The listing builds one solid part. Answer for the finished solid, in the listing's coordinates (mm). A direction names the side the tool comes from. Coordinates: 2 decimals unless noted, no trailing zeros. Order: outer loops, then holes, each group sorted by start corner. A loop starts at its lowest first (then second) coordinate and runs counter-clockwise, first axis right, second up. Notation, with made-up numbers: (-2, 83) -> (41, 83) arc R8 cw to (41, 87) -> close; hole circle Ø4 at (13, -2). An arc over 180 degrees is marked (long way). Write each question's results on one line, items separated by ' | '. Start each with the question number.
(1) A tool of negligible diameter and unlimited length cuts with its end or side. For faces 1 (the face through (-2, -112, 2)), 2 (the face through (-2, 19, 2)), 3 (the face through (25.5, 120, 4)), from which of +Z, -Z, +X, -X, +Y, -Y can it reach the whole face along a straight path? Write none if from no direction.
(2) Determine the mould class of faces 4 (the face through (-31, -1, 4)), 5 (the face through (-2, 64, 2)), 6 (the face through (-31.5, 1, 3)), 7 (the face through (28.5, 1, 3)) for opening direction X: +X half, -X half, draft (parallel to the pull), parting line (faces both ways), or undercut.
(3) The part is cut by section A-A, the plane x = -0.5. Give the vertices of the cut face in (y, z), then the cut area to 3 significant figures.
(4) Straight lines are drawn through the part: L1, parallel to X at y = 24.5, z = 0.5; L2, parallel to Y at x = 19, z = 2.75; L3, parallel to Y at x = 26.5, z = 7.5. For each, find the intervals that lie inside material, in ascending order.
(5) The part is cut by section B-B, the plane y = -84.5. Give the vertices of the cut face in (x, z).
(6) Given pin 1 (2 mm diameter, centred on x = 6.5, z = 2, fed in from -Y); pin 2 (6 mm diameter, centred on x = 0.5, z = 6.5, fed in from +Y); pin 3 (1.5 mm diameter, centred on x = 3, y = 65.5, fed in from +Z), each flat-ended and moving along its own axis, determine where each tip first touches the part or whether it passes through.
```python
from build123d import *

# Parameters (mm, degrees)
F0_W     = 3
F0_H     = 4
F1_DEPTH = 122
F2_W     = 3
F2_H     = 4
F3_DEPTH = 54
F6_DEPTH = 3
F8_DEPTH = 3
F9_R     = 1.5
F10_R    = 1
F11_R    = 2


with BuildPart() as f1:
    # F0 (on Front) → F1 (new body)
    with BuildSketch(Plane.XZ):
        with Locations((-30, 2)):
            Rectangle(F0_W, F0_H)
    extrude(amount=F1_DEPTH)


with BuildPart() as f1b:
    # F0 (on Front) → F1, piece 2 (new body)
    with BuildSketch(Plane.XZ):
        with Locations((27, 2)):
            Rectangle(F0_W, F0_H)
    extrude(amount=F1_DEPTH)


with BuildPart() as f3:
    # F2 (on face) → F3 (new body, through all)
    with BuildSketch(Plane.YZ.offset(-28.5)):
        with Locations((-110.5, 2)):
            Rectangle(F2_W, F2_H)
    extrude(amount=F3_DEPTH)


with BuildPart() as f3b:
    # F2 (on face) → F3, piece 2 (new body, through all)
    with BuildSketch(Plane.YZ.offset(-28.5)):
        with Locations((-65.5, 2)):
            Rectangle(F2_W, F2_H)
    extrude(amount=F3_DEPTH)


with BuildPart() as f3c:
    # F2 (on face) → F3, piece 3 (new body, through all)
    with BuildSketch(Plane.YZ.offset(-28.5)):
        with Locations((-20.5, 2)):
            Rectangle(F2_W, F2_H)
    extrude(amount=F3_DEPTH)


with BuildPart() as f1_1:
    add(f1.part)

    # F4: union F1b, F3, F3b, F3c
    add(f1b.part)
    add(f3.part)
    add(f3b.part)
    add(f3c.part)

    # F5 (on face) → F6 (join, through all)
    with BuildSketch(Plane.YZ.offset(-28.5)):
        Polygon((-122, 7.2), (-122, 4), (-120, 4), (-120, 7.2), (-118, 7.2), (-118, 10.2), (-122, 10.2), align=None)
    extrude(amount=-F6_DEPTH)

    # F7 (on face) → F8 (join, through all)
    with BuildSketch(Plane.YZ.offset(28.5)):
        Polygon((-122, 7.2), (-122, 4), (-120, 4), (-120, 7.2), (-118, 7.2), (-118, 10.2), (-122, 10.2), align=None)
    extrude(amount=-F8_DEPTH)

    # F9
    f9_edges = [f1_1.edges().sort_by_distance(p)[0] for p in [
        (-30, -122, 0),
        (27, -122, 0),
        (27, -122, 10.2),
        (-30, -122, 10.2),
        (27, -120, 4),
        (27, -120, 7.2),
        (-30, -120, 4),
        (-30, -120, 7.2),
    ]]
    fillet(f9_edges, radius=F9_R)

    # F10
    f10_edges = [f1_1.edges().sort_by_distance(p)[0] for p in [
        (-30, -118, 7.2),
        (27, -118, 7.2),
    ]]
    fillet(f10_edges, radius=F10_R)

    # F11
    f11_edges = [f1_1.edges().sort_by_distance(p)[0] for p in [
        (-28.5, -109, 2),
        (-28.5, -64, 2),
        (25.5, -109, 2),
        (25.5, -22, 2),
        (25.5, -67, 2),
        (-28.5, -67, 2),
        (-28.5, -22, 2),
        (-28.5, -19, 2),
        (-28.5, -112, 2),
        (25.5, -112, 2),
        (25.5, -64, 2),
        (25.5, -19, 2),
    ]]
    fillet(f11_edges, radius=F11_R)

    # F12: F1 across plane


with BuildPart() as f1_2:
    add(f1_1.part)
    add(f1_1.part.mirror(Plane.XZ))


solid = f1_2.part
```
Established:
1) face 1: +Z, -Z, -Y | face 2: +Z, -Z | face 3: +Z, -Z, +Y
2) face 4: draft | face 5: undercut | face 6: -X half | face 7: +X half
3) outline: (-112, 0) -> (-109, 0) -> (-109, 4) -> (-112, 4) -> close; (-67, 0) -> (-64, 0) -> (-64, 4) -> (-67, 4) -> close; (-22, 0) -> (-19, 0) -> (-19, 4) -> (-22, 4) -> close; (19, 0) -> (22, 0) -> (22, 4) -> (19, 4) -> close; (64, 0) -> (67, 0) -> (67, 4) -> (64, 4) -> close; (109, 0) -> (112, 0) -> (112, 4) -> (109, 4) -> close | area: 72.0 mm^2
4) L1: x = -31.5 to -28.5, 25.5 to 28.5 | L2: y = -112 to -109, -67 to -64, -22 to -19, 19 to 22, 64 to 67, 109 to 112 | L3: y = -122 to -118.24, 118.24 to 122
5) outline: (-31.5, 0) -> (-28.5, 0) -> (-28.5, 4) -> (-31.5, 4) -> close; (25.5, 0) -> (28.5, 0) -> (28.5, 4) -> (25.5, 4) -> close
6) pin 1: stops at y = -112 | pin 2: stops at y = 112 | pin 3: stops at z = 4
